For this review, use the dimensioned drawing (mm, ordinates from the lowest corner) and the shaded views. A direction names the side the tool comes from. Give positions to 0.01 mm unless a question says otherwise; leave off trailing zeros. Write each loop counter-clockwise with the first axis right and the second up, starting at its lowest first coordinate (ties: lowest second). Pieces come first, ordered by that corner, then holes. Notation, with made-up numbers: M 54,9 L 93,9 A23 cw 93,33 Z; hole C 66.5,75.5 d8. An arc over 180 degrees is marked long. Answer in a Markdown table with one row per item.
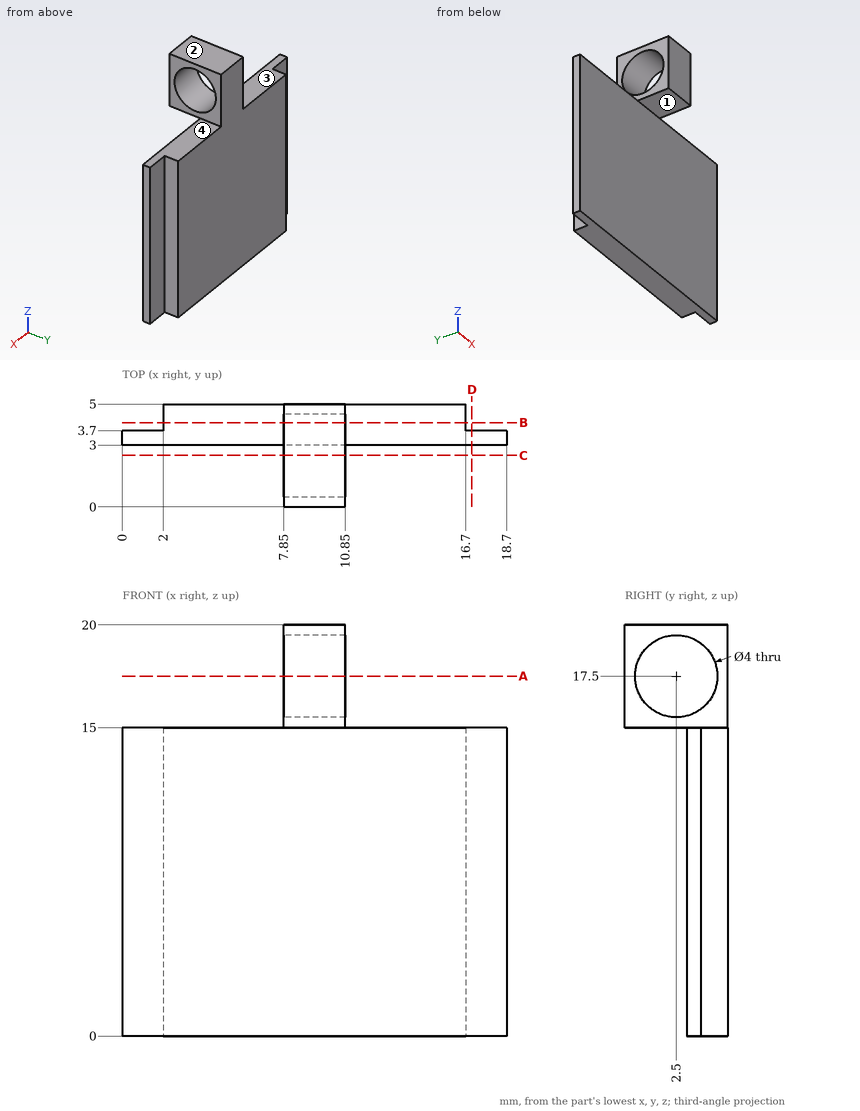
1) For the marked faces 1, 2, 3 and 4, list the 3-axis set-ups (+Z, -Z, +X, -X, +Y, -Y) from which the entire face can be reached by the end or side of a thin tool; tool diameter is ignored.
Geometry says:
| item | result |
|---|---|
| face 1 | -Z, +X, -X, -Y |
| face 2 | +Z, +X, -X, +Y, -Y |
| face 3 | +Z, -X, +Y, -Y |
| face 4 | +Z, +X, +Y, -Y |
2) Add section A-A (z = 17.5). Write out the cut boundary in (x, y), and give its area (3 significant figures).
Geometry says:
| item | result |
|---|---|
| outline | M 7.85,0 L 10.85,0 L 10.85,0.5 L 7.85,0.5 Z; M 7.85,4.5 L 10.85,4.5 L 10.85,5 L 7.85,5 Z |
| area | 3.00 mm^2 |
3) Insertion check: P1, Ø1.4, axis at y = 4.5, z = 4.5, coming from the -X side; P2, Ø1, axis at x = 5, y = 4.5, coming from the +Z side; P3, Ø5, axis at x = 11, z = 2, coming from the -Y side. Each pin has a flat end and moves straight along its axis. Give the tip position at first contact, or say it passes through.
Geometry says:
| item | result |
|---|---|
| P1 | x = 2 |
| P2 | z = 15 |
| P3 | y = 3 |
4) Add section D-D (x = 17). Write out the cut boundary in (y, z), and give its area (3 significant figures).
Geometry says:
| item | result |
|---|---|
| outline | M 3,0 L 3.7,0 L 3.7,15 L 3,15 Z |
| area | 10.5 mm^2 |
5) Add section C-C (y = 2.5). Write out the cut boundary in (x, z), and give its area (3 significant figures).
Geometry says:
| item | result |
|---|---|
| outline | M 7.85,15 L 10.85,15 L 10.85,15.5 L 7.85,15.5 Z; M 7.85,19.5 L 10.85,19.5 L 10.85,20 L 7.85,20 Z |
| area | 3.00 mm^2 |
6) Add section B-B (y = 4.1). Write out the cut boundary in (x, z), and give its area (3 significant figures).
Geometry says:
| item | result |
|---|---|
| outline | M 2,0 L 16.7,0 L 16.7,15 L 10.85,15 L 10.85,16.3 L 7.85,16.3 L 7.85,15 L 2,15 Z; M 7.85,18.7 L 10.85,18.7 L 10.85,20 L 7.85,20 Z |
| area | 228 mm^2 |
7) To check wall thickness, follow probe 1 along Z at (x, y) = (8.6, 2.5); probe 2 along X at (y, z) = (3.95, 9.75); probe 3 along Y at (x, z) = (14.5, 4.5). State the ranges of each line that lie inside material, in increasing order. Write a range as [from, to].
Geometry says:
| item | result |
|---|---|
| probe 1 | [15, 15.5], [19.5, 20] |
| probe 2 | [2, 16.7] |
| probe 3 | [3, 5] |
